Geometry check sheet. Reference: drawing and pictorial views, mm from the part's lowest x, y, z. Round coordinates to 2 decimals unless told otherwise and drop trailing zeros. Write each loop counter-clockwise with the first axis right and the second up, starting at its lowest first coordinate (ties: lowest second). Pieces come first, ordered by that corner, then holes. Notation, with made-up numbers: (-3, -24.75) - (7, -24.75) arc R25 ccw to (7, 11.25) - close; hole circle Ø6 at (27.5, 87). An arc over 180 degrees is marked (long way). Return JSON: item names as keys, results as strings.
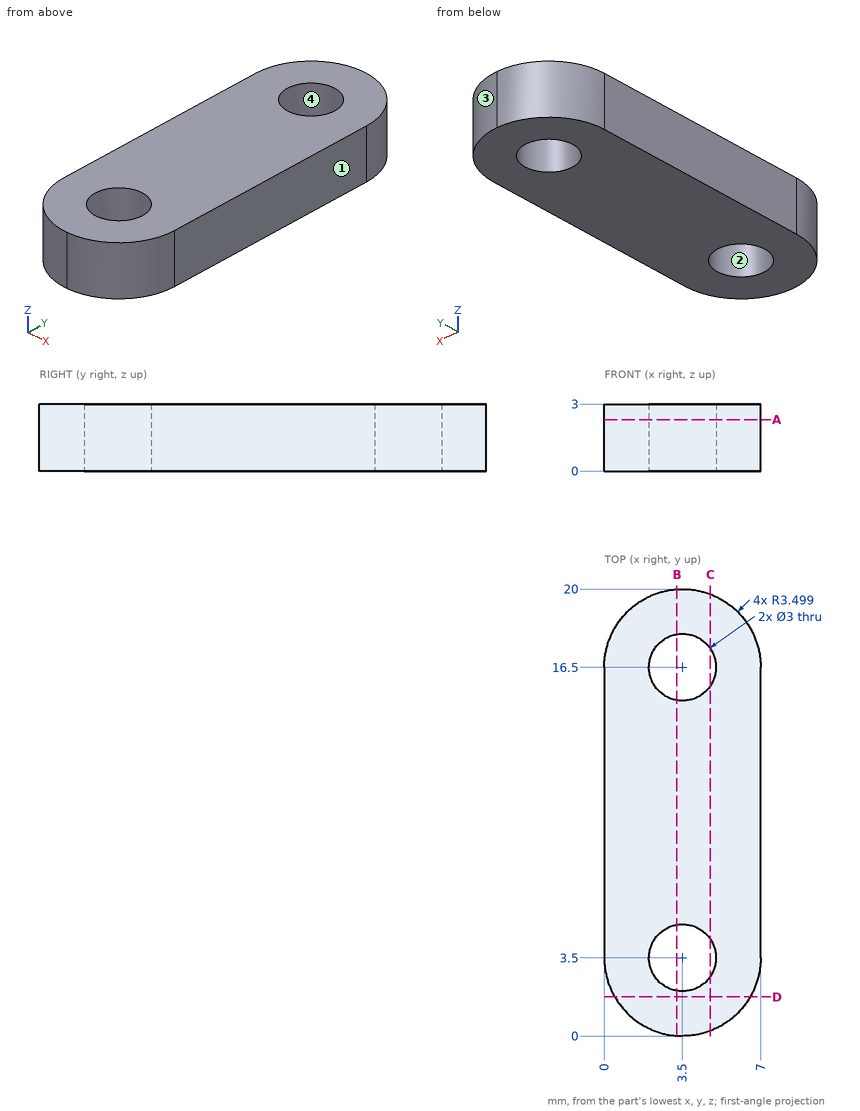
(1) Section check B-B, the plane x = 3.25. Enter the section's corners in (y, z).
Response values:
{"outline": "(0.01, 0) - (2.02, 0) - (2.02, 3) - (0.01, 3) - close; (4.98, 0) - (15.02, 0) - (15.02, 3) - (4.98, 3) - close; (17.98, 0) - (19.99, 0) - (19.99, 3) - (17.98, 3) - close"}
(2) Gauge pin test, flat ends, axial feed: pin 1 (2.5 mm diameter, centred on x = 3.5, y = 16.5, fed in from -Z); pin 2 (1.5 mm diameter, centred on x = 2.5, z = 1, fed in from -Y). Record the tip position at first contact, or that the pin passes through.
Response values:
{"pin 1": "passes through", "pin 2": "stops at y = 0.01"}
(3) Material ranges on line 1 along Y through (x, z) = (3.5, 2); line 2 along X through (y, z) = (3.5, 1.55); line 3 along Y through (x, z) = (2.25, 0.5) (1 decimal), recorded low to high. Write a range as [from, to].
Response values:
{"line 1": "y = [0, 2], [5, 15], [18, 20]", "line 2": "x = [0, 2], [5, 7]", "line 3": "y = [0.2, 2.7], [4.3, 15.7], [17.3, 19.8]"}
(4) Section check A-A, the plane z = 2.3. Give the number of separate pieces and of enclosed holes in the cut face, plus the area to 3 significant figures.
Response values:
{"separate pieces": "1", "enclosed holes": "2", "area": "115 mm^2"}
(5) Section check D-D, the plane y = 1.75. Enter the section's corners in (x, z), plus the area to 3 significant figures.
Response values:
{"outline": "(0.47, 0) - (6.53, 0) - (6.53, 3) - (0.47, 3) - close", "area": "18.2 mm^2"}
(6) Section check C-C, the plane x = 4.75. Enter the section's corners in (y, z).
Response values:
{"outline": "(0.23, 0) - (2.67, 0) - (2.67, 3) - (0.23, 3) - close; (4.33, 0) - (15.67, 0) - (15.67, 3) - (4.33, 3) - close; (17.33, 0) - (19.77, 0) - (19.77, 3) - (17.33, 3) - close"}
(7) Release check for a two-part mould opening along Y. For the marked faces 1, 2, 3 and 4 record: pulls with the +Y half, pulls with the -Y half, needs draft (parallel to the pull), parting line crosses it, or undercut.
Response values:
{"face 1": "needs draft", "face 2": "undercut", "face 3": "pulls with the +Y half", "face 4": "undercut"}
